For this review, take the finished solid that the model builds, in its own axes (mm). A direction names the side the tool comes from. Coordinates: 2 decimals unless noted, no trailing zeros. Write each loop counter-clockwise with the first axis right and the second up, starting at its lowest first coordinate (ties: lowest second). Pieces come first, ordered by that corner, then holes. Notation, with made-up numbers: (82.5, 42) - (106.5, 42) arc R32 ccw to (106.5, 80) - close; hole circle Ø9 at (9.5, -21). An arc over 180 degrees is marked (long way). Write each question's results on one line, items separated by ' | '.
from build123d import *

# Parameters (mm, degrees)
BOSS_EXTRUDE1_DEPTH = 6
BOSS_EXTRUDE2_DEPTH = 3


with BuildPart() as part:
    # Sketch1 → Boss-Extrude1 (new body)
    with BuildSketch(Plane(origin=(0, 0, 0), x_dir=(1, 0, 0), z_dir=(0, 1, 0))):
        with BuildLine():
            Line((-21.042961381, 71.822608989), (-50.715055762, 71.822608989))
            ThreePointArc((-50.715055762, 71.822608989), (-51.215055762, 71.688634393), (-51.581081166, 71.322608989))
            Line((-51.581081166, 71.322608989), (-56.132737248, 63.438909397))
            Line((-56.132737248, 63.438909397), (-15.625279896, 63.438909397))
            Line((-15.625279896, 63.438909397), (-20.176935977, 71.322608989))
            ThreePointArc((-20.176935977, 71.322608989), (-20.542961381, 71.688634393), (-21.042961381, 71.822608989))
        make_face()
    extrude(amount=BOSS_EXTRUDE1_DEPTH)

    # Sketch2 → Boss-Extrude2 (add)
    with BuildSketch(Plane(origin=(0, 6, 0), x_dir=(1, 0, 0), z_dir=(0, 1, 0))):
        with BuildLine():
            Line((-13.893229088, 61.438909397), (-57.864788055, 61.438909397))
            ThreePointArc((-57.864788055, 61.438909397), (-58.730813459, 61.938909397), (-58.730813459, 62.938909397))
            Line((-58.730813459, 62.938909397), (-52.735781704, 73.322608989))
            ThreePointArc((-52.735781704, 73.322608989), (-52.3697563, 73.688634393), (-51.8697563, 73.822608989))
            Line((-51.8697563, 73.822608989), (-19.888260843, 73.822608989))
            ThreePointArc((-19.888260843, 73.822608989), (-19.388260843, 73.688634393), (-19.022235439, 73.322608989))
            Line((-19.022235439, 73.322608989), (-13.027203684, 62.938909397))
            ThreePointArc((-13.027203684, 62.938909397), (-13.027203684, 61.938909397), (-13.893229088, 61.438909397))
        make_face()
    extrude(amount=BOSS_EXTRUDE2_DEPTH)


solid = part.part
Q1. Take a section at C-C on y = 1. State the section outline as (x, z) points, plus the area to 3 significant figures.
Results found:
outline: (-56.13, -63.44) - (-51.58, -71.32) arc R1 ccw to (-50.72, -71.82) - (-21.04, -71.82) arc R1 ccw to (-20.18, -71.32) - (-15.63, -63.44) - close | area: 299 mm2
Q2. Take a section at B-B on z = -65. State the section outline as (x, y) points, plus the area to 3 significant figures.
Results found:
outline: (-57.54, 6) - (-55.23, 6) - (-55.23, 0) - (-16.53, 0) - (-16.53, 6) - (-14.22, 6) - (-14.22, 9) - (-57.54, 9) - close | area: 362 mm2
Q3. Wall thickness on line 1 along Y through (x, z) = (-24.5, -62.75); line 2 along Z through (x, y) = (-45, 1.25); line 3 along Z through (x, y) = (-16.5, 5.25): over which ranges is each line inside the solid? List them lowest first. Write a range as from..to.
Results found:
line 1: 6..9 | line 2: -71.82..-63.44 | line 3: -64.95..-63.44
Q4. For faces 1 (the face through (-36, 3, -63.439)), 2 (the face through (-17.87, 2.96, -67.33)), 3 (the face through (-51.21, 2.96, -71.69)), 4 (the face through (-36, 3, -71.823)), list the 3-axis set-ups (+Z, -Z, +X, -X, +Y, -Y) from which the entire face can be reached by the end or side of a thin tool; tool diameter is ignored.
Results found:
face 1: +Z, +X, -X, -Y | face 2: -Z, +X, -Y | face 3: -Z, -X, -Y | face 4: -Z, +X, -X, -Y
Q5. For pin 1 (1.5 mm diameter, centred on y = 7.5, z = -69.5, fed in from -X); pin 2 (1.8 mm diameter, centred on x = -40, y = 2, fed in from -Z), all flat-tipped, find the tip position at first contact; note any pin that passes through.
Results found:
pin 1: x = -55.38 | pin 2: z = -71.82
Q6. Take a section at A-A on y = 6.75. State the section outline as (x, z) points, plus the area to 3 significant figures.
Results found:
outline: (-58.73, -62.94) - (-52.74, -73.32) arc R1 ccw to (-51.87, -73.82) - (-19.89, -73.82) arc R1 ccw to (-19.02, -73.32) - (-13.03, -62.94) arc R1 ccw to (-13.89, -61.44) - (-57.86, -61.44) arc R1 ccw to start | area: 497 mm2
